Part model, mm, in its own coordinate system. A direction names the side the tool comes from. Round coordinates to 2 decimals unless told otherwise and drop trailing zeros. Write each loop counter-clockwise with the first axis right and the second up, starting at its lowest first coordinate (ties: lowest second). Pieces come first, ordered by that corner, then holes. Notation, with made-up numbers: M 65,-38.75 L 88,-38.75 A25 cw 88,-1.75 Z; hole C 2.25,-13.5 d3. An arc over 180 degrees is marked long. Use a Markdown table: item, result. Add a question column.
1) Slice it at B-B on x = 0. Write the cut outline in (y, z), plus the area to 3 significant figures.
2) Slice it at A-A on z = 0. Write the cut outline in (x, y).
3) Two-plate mould, pull along X, no slides. Class faces 1 (the face through (-16, 21, 0)), 2 (the face through (-15, 20, 0)), 3 (the face through (-15.25, -21.55, -3.38)), 4 (the face through (-15.25, -22.82, 3.38)): released by +X, released by -X, zero draft, split by the parting line, or undercut.
4) Wall check: probe 1 along X at (y, z) = (-22, 0); probe 2 along X at (y, z) = (2, 0); probe 3 along Z at (x, y) = (2, -0.5). Give the ranges that are in metal, low to high.
5) Drop flat-ended pins along their axis: P1, Ø8, axis at y = 5, z = 5, coming from the +X side; P2, Ø5, axis at x = -13, z = 3, coming from the -Y side; P3, Ø1.1, axis at x = -15.5, z = 1, coming from the +Y side; P4, Ø0.7, axis at x = 15.5, z = -0.5, coming from the -Y side. Give the stop position or say it passes through.
6) Which spindle directions (+Z, -Z, +X, -X, +Y, -Y) get a long thin tool onto all of the face, cutting with end or side? Do faces 5 (the face through (-12, -15, -2)), 6 (the face through (16, 21, 0)), 7 (the face through (13, -20.7, -8)), 8 (the face through (17.084, -19.93, -3.794)), 9 (the face through (-10.5, -25, 10.5)). Say none if no direction does.
```python
from build123d import *

# Parameters (mm, degrees)
SKETCH2_W          = 2
SKETCH2_H          = 2
REVOLVE2_ANGLE     = 20
SKETCH3_W          = 2.2
SKETCH3_H          = 6.8
CUT_REVOLVE1_ANGLE = 25
SKETCH4_W          = 4.7
SKETCH4_H          = 2.5
CUT_REVOLVE2_ANGLE = 45


with BuildPart() as part:
    # Sketch1 → Revolve1 (revolve)
    with BuildSketch(Plane.XY, mode=Mode.PRIVATE) as revolve1_sk:
        Polygon((12, 25), (12, -15), (14.5, -15), (14.5, -25), (17.5, -25), (17.5, -15), (14, -7), (14, 25), align=None)
    revolve(revolve1_sk.sketch.rotate(Axis((0, 40.467735012, 0), (0, -1, 0)), 90), axis=Axis((0, 40.467735012, 0), (0, -1, 0)))

    # Sketch2 → Revolve2 (revolve, symmetric)
    with BuildSketch(Plane.XY) as revolve2_sk:
        with Locations((15, 21)):
            Rectangle(SKETCH2_W, SKETCH2_H)
        with Locations((-15, 21)):
            Rectangle(SKETCH2_W, SKETCH2_H)
    revolve(axis=Axis((0, 45.306661743, 0), (0, -1, 0)), revolution_arc=REVOLVE2_ANGLE / 2)
    revolve(revolve2_sk.sketch, axis=Axis((0, 45.306661743, 0), (0, 1, 0)), revolution_arc=REVOLVE2_ANGLE / 2)

    # Sketch3 → Cut-Revolve1 (revolve, symmetric, cut)
    with BuildSketch(Plane.XY) as cut_revolve1_sk:
        with Locations((-15.6, -21.6)):
            Rectangle(SKETCH3_W, SKETCH3_H)
        with Locations((15.6, -21.6)):
            Rectangle(SKETCH3_W, SKETCH3_H)
    revolve(axis=Axis((0, -11.020729768, 0), (0, -1, 0)), revolution_arc=CUT_REVOLVE1_ANGLE / 2, mode=Mode.SUBTRACT)
    revolve(cut_revolve1_sk.sketch, axis=Axis((0, -11.020729768, 0), (0, 1, 0)), revolution_arc=CUT_REVOLVE1_ANGLE / 2, mode=Mode.SUBTRACT)

    # Sketch4 → Cut-Revolve2 (revolve, cut)
    with BuildSketch(Plane.XY):
        with Locations((-14.35, -19.45)):
            Rectangle(SKETCH4_W, SKETCH4_H)
        with Locations((14.35, -19.45)):
            Rectangle(SKETCH4_W, SKETCH4_H)
    revolve(axis=Axis((0, -42.004114959, 0), (0, 1, 0)), revolution_arc=CUT_REVOLVE2_ANGLE, mode=Mode.SUBTRACT)


solid = part.part
```
Entries:
| question | item | result |
|---|---|---|
| 1 | outline | M -25,-17.5 L -15,-17.5 L -7,-14 L 25,-14 L 25,-12 L -15,-12 L -15,-14.5 L -25,-14.5 Z; M -25,14.5 L -15,14.5 L -15,12 L 25,12 L 25,14 L -7,14 L -15,17.5 L -25,17.5 Z |
| 1 | area | 248 mm^2 |
| 2 | outline | M -17.5,-25 L -16.7,-25 L -16.7,-18.2 L -14.5,-18.2 L -14.5,-15 L -12,-15 L -12,25 L -14,25 L -14,22 L -16,22 L -16,20 L -14,20 L -14,-7 L -17.5,-15 Z; M 12,-15 L 14.5,-15 L 14.5,-18.2 L 16.7,-18.2 L 16.7,-25 L 17.5,-25 L 17.5,-15 L 14,-7 L 14,20 L 16,20 L 16,22 L 14,22 L 14,25 L 12,25 Z |
| 3 | face 1 | released by -X |
| 3 | face 2 | zero draft |
| 3 | face 3 | undercut |
| 3 | face 4 | undercut |
| 4 | probe 1 | x = -17.5 to -16.7, 16.7 to 17.5 |
| 4 | probe 2 | x = -14 to -12, 12 to 14 |
| 4 | probe 3 | z = -13.86 to -11.83, 11.83 to 13.86 |
| 5 | P1 | stops at x = 13.96 |
| 5 | P2 | stops at y = -25 |
| 5 | P3 | stops at y = 22 |
| 5 | P4 | stops at y = -18.2 |
| 6 | face 5 | -Y |
| 6 | face 6 | +X, +Y |
| 6 | face 7 | none |
| 6 | face 8 | +Y, -Y |
| 6 | face 9 | +Z, -Z, +X, -X, -Y |
